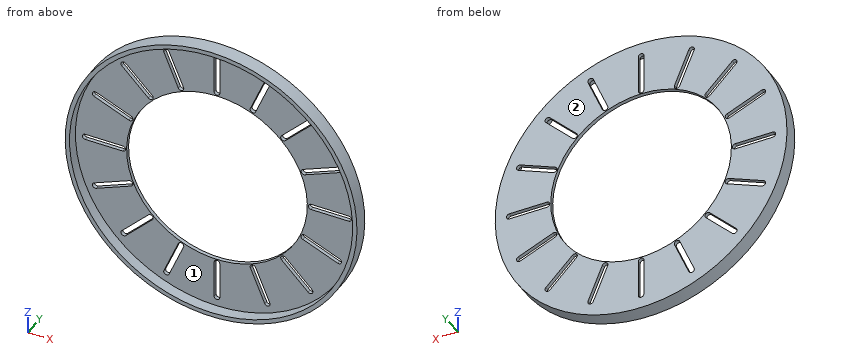
```python
from build123d import *

# Parameters (mm, degrees)
SKETCH1_R           = 38.75
SKETCH1_R_2         = 37.6
BOSS_EXTRUDE1_DEPTH = 3
SKETCH2_R           = 38.75
SKETCH2_R_2         = 24
BOSS_EXTRUDE2_DEPTH = 1
CUT_EXTRUDE3_DEPTH  = 1


with BuildPart() as part:
    # Sketch1 → Boss-Extrude1 (new body)
    with BuildSketch(Plane(origin=(0, 0, 0), x_dir=(1, 0, 0), z_dir=(0, 1, 0))):
        with Locations(Location((0, 0, 0), (0, 0, 270))):
            Circle(SKETCH1_R)
        with Locations(Location((0, 0, 0), (0, 0, 270))):
            Circle(SKETCH1_R_2, mode=Mode.SUBTRACT)
    extrude(amount=BOSS_EXTRUDE1_DEPTH)

    # Sketch2 → Boss-Extrude2 (add)
    with BuildSketch(Plane(origin=(0, 3, 0), x_dir=(1, 0, 0), z_dir=(0, 1, 0))):
        with Locations(Location((0, 0, 0), (0, 0, 270))):
            Circle(SKETCH2_R)
        with Locations(Location((0, 0, 0), (0, 0, 270))):
            Circle(SKETCH2_R_2, mode=Mode.SUBTRACT)
    extrude(amount=BOSS_EXTRUDE2_DEPTH)

    # Sketch4 → Cut-Extrude3 (cut)
    with BuildSketch(Plane(origin=(0, 4, 0), x_dir=(1, 0, 0), z_dir=(0, 1, 0))):
        with BuildLine():
            Line((-0.75, 25), (-0.75, 35))
            ThreePointArc((-0.75, 35), (0, 35.75), (0.75, 35))
            Line((0.75, 35), (0.75, 25))
            ThreePointArc((0.75, 25), (0, 24.25), (-0.75, 25))
        make_face()
        with BuildLine():
            Line((8.87417616, 23.384000887), (12.701010483, 32.622796212))
            ThreePointArc((12.701010483, 32.622796212), (13.680932707, 33.028693287), (14.086829782, 32.048771064))
            Line((14.086829782, 32.048771064), (10.259995459, 22.809975739))
            ThreePointArc((10.259995459, 22.809975739), (9.280073235, 22.404078663), (8.87417616, 23.384000887))
        make_face()
        with BuildLine():
            Line((17.147339444, 18.207999616), (24.218407256, 25.279067427))
            ThreePointArc((24.218407256, 25.279067427), (25.279067427, 25.279067427), (25.279067427, 24.218407256))
            Line((25.279067427, 24.218407256), (18.207999616, 17.147339444))
            ThreePointArc((18.207999616, 17.147339444), (17.147339444, 17.147339444), (17.147339444, 18.207999616))
        make_face()
        with BuildLine():
            Line((22.809975739, 10.259995459), (32.048771064, 14.086829782))
            ThreePointArc((32.048771064, 14.086829782), (33.028693287, 13.680932707), (32.622796212, 12.701010483))
            Line((32.622796212, 12.701010483), (23.384000887, 8.87417616))
            ThreePointArc((23.384000887, 8.87417616), (22.404078663, 9.280073235), (22.809975739, 10.259995459))
        make_face()
        with BuildLine():
            Line((25, 0.75), (35, 0.75))
            ThreePointArc((35, 0.75), (35.75, 0), (35, -0.75))
            Line((35, -0.75), (25, -0.75))
            ThreePointArc((25, -0.75), (24.25, 0), (25, 0.75))
        make_face()
        with BuildLine():
            Line((23.384000887, -8.87417616), (32.622796212, -12.701010483))
            ThreePointArc((32.622796212, -12.701010483), (33.028693287, -13.680932707), (32.048771064, -14.086829782))
            Line((32.048771064, -14.086829782), (22.809975739, -10.259995459))
            ThreePointArc((22.809975739, -10.259995459), (22.404078663, -9.280073235), (23.384000887, -8.87417616))
        make_face()
        with BuildLine():
            Line((18.207999616, -17.147339444), (25.279067427, -24.218407256))
            ThreePointArc((25.279067427, -24.218407256), (25.279067427, -25.279067427), (24.218407256, -25.279067427))
            Line((24.218407256, -25.279067427), (17.147339444, -18.207999616))
            ThreePointArc((17.147339444, -18.207999616), (17.147339444, -17.147339444), (18.207999616, -17.147339444))
        make_face()
        with BuildLine():
            Line((10.259995459, -22.809975739), (14.086829782, -32.048771064))
            ThreePointArc((14.086829782, -32.048771064), (13.680932707, -33.028693287), (12.701010483, -32.622796212))
            Line((12.701010483, -32.622796212), (8.87417616, -23.384000887))
            ThreePointArc((8.87417616, -23.384000887), (9.280073235, -22.404078663), (10.259995459, -22.809975739))
        make_face()
        with BuildLine():
            Line((0.75, -25), (0.75, -35))
            ThreePointArc((0.75, -35), (0, -35.75), (-0.75, -35))
            Line((-0.75, -35), (-0.75, -25))
            ThreePointArc((-0.75, -25), (0, -24.25), (0.75, -25))
        make_face()
        with BuildLine():
            Line((-8.87417616, -23.384000887), (-12.701010483, -32.622796212))
            ThreePointArc((-12.701010483, -32.622796212), (-13.680932707, -33.028693287), (-14.086829782, -32.048771064))
            Line((-14.086829782, -32.048771064), (-10.259995459, -22.809975739))
            ThreePointArc((-10.259995459, -22.809975739), (-9.280073235, -22.404078663), (-8.87417616, -23.384000887))
        make_face()
        with BuildLine():
            Line((-17.147339444, -18.207999616), (-24.218407256, -25.279067427))
            ThreePointArc((-24.218407256, -25.279067427), (-25.279067427, -25.279067427), (-25.279067427, -24.218407256))
            Line((-25.279067427, -24.218407256), (-18.207999616, -17.147339444))
            ThreePointArc((-18.207999616, -17.147339444), (-17.147339444, -17.147339444), (-17.147339444, -18.207999616))
        make_face()
        with BuildLine():
            Line((-22.809975739, -10.259995459), (-32.048771064, -14.086829782))
            ThreePointArc((-32.048771064, -14.086829782), (-33.028693287, -13.680932707), (-32.622796212, -12.701010483))
            Line((-32.622796212, -12.701010483), (-23.384000887, -8.87417616))
            ThreePointArc((-23.384000887, -8.87417616), (-22.404078663, -9.280073235), (-22.809975739, -10.259995459))
        make_face()
        with BuildLine():
            Line((-25, -0.75), (-35, -0.75))
            ThreePointArc((-35, -0.75), (-35.75, 0), (-35, 0.75))
            Line((-35, 0.75), (-25, 0.75))
            ThreePointArc((-25, 0.75), (-24.25, 0), (-25, -0.75))
        make_face()
        with BuildLine():
            Line((-23.384000887, 8.87417616), (-32.622796212, 12.701010483))
            ThreePointArc((-32.622796212, 12.701010483), (-33.028693287, 13.680932707), (-32.048771064, 14.086829782))
            Line((-32.048771064, 14.086829782), (-22.809975739, 10.259995459))
            ThreePointArc((-22.809975739, 10.259995459), (-22.404078663, 9.280073235), (-23.384000887, 8.87417616))
        make_face()
        with BuildLine():
            Line((-18.207999616, 17.147339444), (-25.279067427, 24.218407256))
            ThreePointArc((-25.279067427, 24.218407256), (-25.279067427, 25.279067427), (-24.218407256, 25.279067427))
            Line((-24.218407256, 25.279067427), (-17.147339444, 18.207999616))
            ThreePointArc((-17.147339444, 18.207999616), (-17.147339444, 17.147339444), (-18.207999616, 17.147339444))
        make_face()
        with BuildLine():
            Line((-10.259995459, 22.809975739), (-14.086829782, 32.048771064))
            ThreePointArc((-14.086829782, 32.048771064), (-13.680932707, 33.028693287), (-12.701010483, 32.622796212))
            Line((-12.701010483, 32.622796212), (-8.87417616, 23.384000887))
            ThreePointArc((-8.87417616, 23.384000887), (-9.280073235, 22.404078663), (-10.259995459, 22.809975739))
        make_face()
    extrude(amount=-CUT_EXTRUDE3_DEPTH, mode=Mode.SUBTRACT)


solid = part.part
```
For this review, take the finished solid that the model builds, in its own axes (mm). Face numbers are marked on the shaded views. Give positions to 0.01 mm unless a question says otherwise; leave off trailing zeros. Write each loop counter-clockwise with the first axis right and the second up, starting at its lowest first coordinate (ties: lowest second). Pieces come first, ordered by that corner, then holes.
Item 1: Wall thickness on probe 1 along Z at (x, y) = (-1, 2.7); probe 2 along X at (y, z) = (1, 0); probe 3 along Y at (x, z) = (15, -19): over which ranges is each line inside the solid? List them lowest first.
Item 2: Take a section at C-C (y = 1.1). Give the boundary of the cut face in (x, z), and give its area (3 significant figures).
Item 3: The part is to be moulded in two halves that separate along Z. For the marked faces 1 and 2, say which applies: +Z half, -Z half, draft (parallel to the pull), parting line (faces both ways), or undercut.
Item 4: Take a section at B-B (z = 5). Give the boundary of the cut face in (x, y), and give its area (3 significant figures).
Item 5: Take a section at A-A (x = 31). Give the boundary of the cut face in (y, z).
Item 6: Insertion check: P1, Ø0.5, axis at y = 3.5, z = -28.5, coming from the -X side; P2, Ø1.1, axis at y = 3.5, z = -30, coming from the +X side; P3, Ø0.5, axis at y = 3.5, z = 32.5, coming from the -X side. Each pin has a flat end and moves straight along its axis. Give the tip position at first contact, or say it passes through.
Established:
1. probe 1: z = -38.74 to -37.59, 37.59 to 38.74
1. probe 2: x = -38.75 to -37.6, 37.6 to 38.75
1. probe 3: y = 3 to 4
2. outline: circle Ø77.5 at (0, 0); hole circle Ø75.2 at (0, 0)
2. area: 276 mm2
3. face 1: undercut
3. face 2: draft
4. outline: (-38.43, 0) - (-37.27, 0) - (-37.27, 3) - (-23.47, 3) - (-23.47, 4) - (-38.43, 4) - close; (23.47, 3) - (37.27, 3) - (37.27, 0) - (38.43, 0) - (38.43, 4) - (23.47, 4) - close
4. area: 36.9 mm2
5. outline: (0, -23.25) - (4, -23.25) - (4, -13.65) - (3, -13.65) - (3, -21.28) - (0, -21.28) - close; (0, 21.28) - (3, 21.28) - (3, 13.65) - (4, 13.65) - (4, 23.25) - (0, 23.25) - close; (3, -12.03) - (4, -12.03) - (4, -0.75) - (3, -0.75) - close; (3, 0.75) - (4, 0.75) - (4, 12.03) - (3, 12.03) - close
6. P1: stops at x = -26.52
6. P2: stops at x = 25.18
6. P3: stops at x = -21.48
